from build123d import *

# Parameters (mm, degrees)
SKETCH012_W     = 266
SKETCH012_H     = 48
PAD009_DEPTH    = 4
SKETCH022_W     = 40
SKETCH022_H     = 30
SKETCH022_W_2   = 30
SKETCH022_H_2   = 20
POCKET005_DEPTH = 4.001
SKETCH038_R     = 1.65
HOLE003_DEPTH   = 25


with BuildPart() as part:
    # Sketch012 (on DatumPlane) → Pad009 (new body)
    with BuildSketch(Plane(origin=(0, -79, -4), x_dir=(-1, 0, 0), z_dir=(0, 1, 0))):
        with Locations((0, 20)):
            Rectangle(SKETCH012_W, SKETCH012_H)
    extrude(amount=PAD009_DEPTH)

    # Sketch022 (on Face5 of Pad009) → Pocket005 (cut, through all)
    with BuildSketch(Plane(origin=(0, -79, -4), x_dir=(-1, 0, 0), z_dir=(0, -1, 0))):
        Polygon((-145, 26), (-100, 26), (-100, -4), (-125, -4), (-125, -19.5), (-155, -19.5), (-155, 0.5), (-145, 0.5), align=None)
        with Locations((-40, 11)):
            Rectangle(SKETCH022_W, SKETCH022_H)
        with Locations((40, 11)):
            Rectangle(SKETCH022_W, SKETCH022_H)
        Polygon((100, 26), (145, 26), (145, 0.5), (155, 0.5), (155, -19.5), (125, -19.5), (125, -4), (100, -4), align=None)
        with Locations((-140, -41.5)):
            Rectangle(SKETCH022_W_2, SKETCH022_H_2)
        with Locations((140, -41.5)):
            Rectangle(SKETCH022_W_2, SKETCH022_H_2)
    extrude(amount=-POCKET005_DEPTH, mode=Mode.SUBTRACT)

    # Sketch038 (on Face2 of Pocket005) → Hole003 (cut)
    with BuildSketch(Plane(origin=(0, -79, -4), x_dir=(-1, 0, 0), z_dir=(0, -1, 0))):
        with Locations((-39.5, -31)):
            Circle(SKETCH038_R)
    extrude(amount=-HOLE003_DEPTH, mode=Mode.SUBTRACT)


solid = part.part
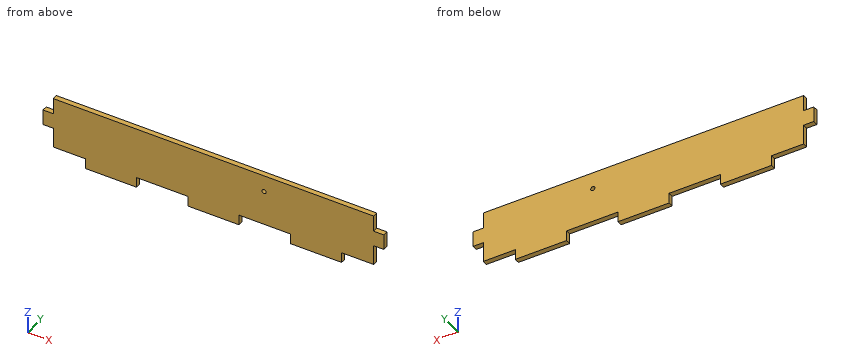
Design review of the part built by this model. Coordinates are the model's own, in mm. Coordinates: 2 decimals unless noted, no trailing zeros. Loops run counter-clockwise (first coordinate to the right, second up) from the corner with the lowest first, then second, coordinate; pieces in that order, holes last.
Item 1: Clearance check with flat-ended pins moving along their axes: pin 1 (1 mm diameter, centred on y = -76.5, z = -1, fed in from +X); pin 2 (1.2 mm diameter, centred on y = -77, z = 7.5, fed in from +X); pin 3 (2 mm diameter, centred on y = -76.5, z = 7, fed in from -X); pin 4 (4.5 mm diameter, centred on x = 39.5, z = 27, fed in from -Y). State where each tip first meets the part, or that it passes through.
Completed:
pin 1: stops at x = 100
pin 2: stops at x = 125
pin 3: stops at x = -125
pin 4: stops at y = -79
Item 2: Add section B-B (x = 106). Write out the cut boundary in (y, z), and give its area (3 significant figures).
Completed:
outline: (-79, 0) - (-75, 0) - (-75, 40) - (-79, 40) - close
area: 160 mm2
Item 3: Add section A-A (y = -77.4). Write out the cut boundary in (x, z).
Completed:
outline: (-133, 15.5) - (-125, 15.5) - (-125, 0) - (-100, 0) - (-100, -8) - (-60, -8) - (-60, 0) - (-20, 0) - (-20, -8) - (20, -8) - (20, 0) - (60, 0) - (60, -8) - (100, -8) - (100, 0) - (125, 0) - (125, 15.5) - (133, 15.5) - (133, 27.5) - (125, 27.5) - (125, 40) - (-125, 40) - (-125, 27.5) - (-133, 27.5) - close; hole circle Ø3.3 at (39.5, 27)
Item 4: Wall thickness on L1, parallel to X at y = -75.85, z = -1; L2, parallel to Z at x = 39.5, y = -77; L3, parallel to X at y = -77.6, z = 27: over which ranges is each line inside the solid? List them lowest first.
Completed:
L1: x = -100 to -60, -20 to 20, 60 to 100
L2: z = 0 to 25.35, 28.65 to 40
L3: x = -133 to 37.85, 41.15 to 133
